from build123d import *

# Parameters (mm, degrees)
F0_W     = 76.2
F0_H     = 25.4
F1_DEPTH = 5.08
F2_W     = 19.28169
F2_H     = 5.94669
F3_DEPTH = 76.2
F5_DEPTH = 6.35


with BuildPart() as f1:
    # F0 (on Top) → F1 (new body)
    with BuildSketch(Plane.XY):
        Rectangle(F0_W, F0_H)
    extrude(amount=F1_DEPTH)

    # F2 (on face) → F3 (join)
    with BuildSketch(Plane.XY.offset(5.08)):
        Rectangle(F2_W, F2_H)
    extrude(amount=F3_DEPTH)

    # F4 (on face) → F5 (join)
    with BuildSketch(Plane(origin=(0, 2.973345, 0), x_dir=(-1, 0, 0), z_dir=(0, 1, 0))):
        Polygon((-4.838744, 81.28), (4.681972, 81.28), (4.681972, 91.884151), (9.640845, 91.884151), (9.640845, 108.11457), (-11.076658, 108.11457), (-11.076658, 92.657104), (-4.838744, 92.657104), align=None)
    extrude(amount=-F5_DEPTH)


solid = f1.part
Source: CAD feature listing. Evaluate the final solid. Frame: model axes, mm. A direction names the side the tool comes from. Round coordinates to 2 decimals unless told otherwise and drop trailing zeros. Write each loop counter-clockwise with the first axis right and the second up, starting at its lowest first coordinate (ties: lowest second). Pieces come first, ordered by that corner, then holes. Notation, with made-up numbers: M -18.75,-37 L 33.25,-37 A30 cw 33.25,-11 Z; hole C 29,41 d9. An arc over 180 degrees is marked long. One line per item, written item: value. Start each with the question number.
Item 1: Pin query (flat end, axial travel): pin 1 (9.5 mm diameter, centred on x = -3, z = 57.5, fed in from -Y); pin 2 (1.9 mm diameter, centred on y = -0.5, z = 88, fed in from +X); pin 3 (1.8 mm diameter, centred on y = 0, z = 62, fed in from +X); pin 4 (8 mm diameter, centred on x = 25, y = 4, fed in from -Z). Return the tip coordinate at first contact, or that it passes through.
Item 2: Section query A-A (x = -8.5). Return the cut outline in (y, z), plus the area to 3 significant figures.
Item 3: Ray query, L1, parallel to X at y = 0.5, z = 13; L2, parallel to Z at x = -32.5, y = -0.25; L3, parallel to Y at x = -3, z = 101.5. Return the intervals inside material, ascending. Write a range as from..to.
Item 4: Section query D-D (y = -5.5). Return the cut outline in (x, z), plus the area to 3 significant figures.
Item 5: Set-up query: faces 1 (the flat face through (-9.641, 0, 100)), 2 (the flat face through (8, 0, 92.657)), 3 (the flat face through (1, 2.973, 57)), 4 (the flat face through (1, -3.377, 98)). Return all of +Z, -Z, +X, -X, +Y, -Y with unobstructed straight access to the full face (end or side cutting, diameter ignored); none if empty.
Item 6: Mould query, pull axis Z, two halves, no side actions, for faces 5 (the flat face through (-9.641, 0, 43)), 6 (the flat face through (-4.682, 0, 87)), 7 (the flat face through (-1, 0, 0)), 8 (the flat face through (-7, 0, 81.28)). Classes: pulls with the +Z half, pulls with the -Z half, needs draft (parallel to the pull), parting line crosses it, or undercut.
Item 7: Section query C-C (z = 22.5). Return the cut outline in (x, y).
Item 8: Section query B-B (x = 7). Return the cut outline in (y, z), plus the area to 3 significant figures.
Result set:
1. pin 1: stops at y = -2.97
1. pin 2: stops at x = 4.84
1. pin 3: stops at x = 9.64
1. pin 4: stops at z = 0
2. outline: M -12.7,0 L 12.7,0 L 12.7,5.08 L 2.97,5.08 L 2.97,81.28 L -2.97,81.28 L -2.97,5.08 L -12.7,5.08 Z; M -3.38,91.88 L 2.97,91.88 L 2.97,108.11 L -3.38,108.11 Z
2. area: 685 mm²
3. L1: x = -9.64..9.64
3. L2: z = 0..5.08
3. L3: y = -3.38..2.97
4. outline: M -38.1,0 L 38.1,0 L 38.1,5.08 L -38.1,5.08 Z
4. area: 387 mm²
5. face 1: +Z, -X, +Y, -Y
5. face 2: +X, +Y, -Y
5. face 3: +Z, +X, -X, +Y
5. face 4: +Z, +X, -X, -Y
6. face 5: needs draft
6. face 6: undercut
6. face 7: pulls with the -Z half
6. face 8: undercut
7. outline: M -9.64,-2.97 L 9.64,-2.97 L 9.64,2.97 L -9.64,2.97 Z
8. outline: M -12.7,0 L 12.7,0 L 12.7,5.08 L 2.97,5.08 L 2.97,81.28 L -2.97,81.28 L -2.97,5.08 L -12.7,5.08 Z; M -3.38,92.66 L 2.97,92.66 L 2.97,108.11 L -3.38,108.11 Z
8. area: 680 mm²
